The model under review builds one solid part; all positions refer to its coordinate system, in mm. A direction names the side the tool comes from. Coordinates: 2 decimals unless noted, no trailing zeros. Order: outer loops, then holes, each group sorted by start corner. A loop starts at its lowest first (then second) coordinate and runs counter-clockwise, first axis right, second up. Notation, with made-up numbers: M -30.5,70.25 L 28.5,70.25 A23 cw 28.5,98.25 Z; hole C 61,24.25 d4. An arc over 180 degrees is marked long. One line per item, written item: value.
Autodesk Inventor part; units mm, degrees
ref_plane "YZ Plane" through (0, 0, 0) normal (1, 0, 0) x (0, 1, 0)
ref_plane "XZ Plane" through (0, 0, 0) normal (0, 1, 0) x (-1, 0, 0)
ref_plane "XY Plane" through (0, 0, 0) normal (0, 0, 1) x (1, 0, 0)
sketch "Sketch1" plane through (0, 0, 0) normal (0, 1, 0) x (-1, 0, 0)
  line L0 (76.2, -76.2) -> (-76.2, -76.2)
  line L1 (-76.2, -76.2) -> (-76.2, 76.2)
  line L2 (76.2, 76.2) -> (76.2, -76.2)
  line L3 (-22.225, -25.4) -> (22.225, -25.4)
  line L4 (22.225, -25.4) -> (22.225, -69.85)
  line L5 (22.225, -69.85) -> (-22.225, -69.85)
  line L6 (-22.225, -69.85) -> (-22.225, -25.4)
  line L7 (-19.05, 56.2) -> (19.05, 56.2)
  line L8 (-76.2, 76.2) -> (-39.05, 76.2)
  line L9 (39.05, 76.2) -> (76.2, 76.2)
  line L10 (19.05, 56.2) -> (39.05, 76.2)
  line L11 (-19.05, 56.2) -> (-39.05, 76.2)
  point P0 (0, 0)
  dimension "d0" = 152.4
  dimension "d2" = 152.4
  dimension "d3" = 76.2
  dimension "d4" = 76.2
  dimension "d5" = 44.45
  dimension "d6" = 44.45
  dimension "d7" = 22.225
  dimension "d26" = 56.2
  dimension "d31" = 45
  dimension "d32" = 45
  dimension "d33" = 38.1
  dimension "d34" = 57.15
  dimension "d56" = 6.35
extrude "Extrusion1" add sketch "Sketch1" along normal blind 6.35
chamfer "Chamfer2" distance 3.175 angle 45 1 edges at (76.2, 3.175, 76.2)
chamfer "Chamfer3" distance 3.175 angle 45 3 edges at (76.2, 3.175, -76.2) (-76.2, 3.175, -76.2) (-76.2, 3.175, 76.2)
sketch "Sketch3" plane through (0, 6.35, 0) normal (0, 1, 0) x (1, 0, 0)
  line L0 (-18.415, 21.59) -> (18.415, 21.59)
  line L1 (21.59, 18.415) -> (21.59, -18.415)
  line L2 (18.415, -21.59) -> (-18.415, -21.59)
  line L3 (-21.59, -18.415) -> (-21.59, 18.415)
  line L4 (-21.59, 18.415) -> (-18.415, 21.59)
  line L5 (18.415, 21.59) -> (21.59, 18.415)
  line L6 (21.59, -18.415) -> (18.415, -21.59)
  line L7 (-18.415, -21.59) -> (-21.59, -18.415)
  point P0 (0, 0)
  point P1 (-21.59, 21.59)
  point P2 (21.59, -21.59)
  point P3 (21.59, 21.59)
  point P4 (-21.59, -21.59)
  dimension "d41" = 43.18
  dimension "d43" = 43.18
  dimension "d44" = 21.59
  dimension "d45" = 21.59
  dimension "d46" = 3.175
  dimension "d47" = 3.175
  dimension "d48" = 3.175
  dimension "d49" = 3.175
  dimension "d50" = 3.175
  dimension "d51" = 3.175
  dimension "d52" = 3.175
  dimension "d53" = 3.175
extrude "Extrusion2" cut sketch "Sketch3" against normal through all
chamfer "Chamfer4" distance 3.175 angle 45 4 edges at (-22.225, 3.175, -69.85) (-22.225, 3.175, -25.4) (22.225, 3.175, -69.85) (22.225, 3.175, -25.4)
sketch "Sketch4" plane through (0, 6.35, 0) normal (0, 1, 0) x (1, 0, 0)
  line L0 (73.025, 76.2) -> (-73.025, 76.2)
  line L1 (-76.2, 73.025) -> (-76.2, -73.025)
  line L2 (-66.675, 69.85) -> (-43.815, 69.85)
  line L3 (-43.815, 69.85) -> (-43.815, 57.785)
  line L4 (-43.815, 57.785) -> (-66.675, 57.785)
  line L5 (-66.675, 57.785) -> (-66.675, 69.85)
  point P0 (0, 0)
  dimension "d60" = 12.065
  dimension "d62" = 22.86
  dimension "d65" = 9.525
  dimension "d66" = 6.35
extrude "Extrusion3" cut sketch "Sketch4" against normal through all
equation "\"d34\" = -0.5 * d33 + 0.5 * d0"
properties part number "carousel_base"
(1) We need section B-B, the plane y = 3.5. Count the separate pieces of the cut face and the enclosed holes in it, plus the area to 3 significant figures.
Geometry results:
separate pieces: 1
enclosed holes: 3
area: 18,000 mm2
(2) For L1, parallel to X at y = 0.5, z = -63.5 (3 decimals); L2, parallel to Z at x = 10, y = 1.25; L3, parallel to Z at x = -55.5, y = 1.75 (3 decimals), list the stretches that pass through material, from the lowest coordinate up.
Geometry results:
L1: x = -76.2 to -66.675, -43.815 to -22.225, 22.225 to 76.2
L2: z = -76.2 to -69.85, -25.4 to -21.59, 21.59 to 56.2
L3: z = -76.2 to -69.85, -57.785 to 76.2
(3) Mouldability with a two-part tool opening along Z and no side actions: class faces 1 (the flat face through (-1, 3, -76.2)), 2 (the flat face through (0, 3, -69.85)), 3 (the flat face through (56, 3, 76.2)) as +Z half, -Z half, draft (parallel to the pull), parting line (faces both ways), or undercut.
Geometry results:
face 1: -Z half
face 2: undercut
face 3: +Z half
(4) We need section D-D, the plane z = 5. State the section outline as (x, y) points.
Geometry results:
outline: M -76.2,0 L -21.59,0 L -21.59,6.35 L -76.2,6.35 Z; M 21.59,0 L 76.2,0 L 76.2,6.35 L 21.59,6.35 Z
(5) Insertion check: pin 1 Ø1.9 at (x, y) = (8.5, 2) entering from +Z. The pin has a flat end and moves straight along its axis. Give the tip position at first contact, or say it passes through.
Geometry results:
pin 1: stops at z = 56.2
(6) We need section C-C, the plane x = 30.5. State the section outline as (y, z) points, plus the area to 3 significant figures.
Geometry results:
outline: M 0,-76.2 L 6.35,-76.2 L 6.35,67.65 L 0,67.65 Z
area: 913 mm2
(7) We need section A-A, the plane z = 63.5. State the section outline as (x, y) points, plus the area to 3 significant figures.
Geometry results:
outline: M -76.2,0 L -26.35,0 L -26.35,6.35 L -76.2,6.35 Z; M 26.35,0 L 76.2,0 L 76.2,6.35 L 26.35,6.35 Z
area: 633 mm2
(8) Tool access review of faces 4 (the flat face through (-66.675, 3, -64)), 5 (the flat face through (-56, 3, 76.2)), 6 (the flat face through (0, 3, 56.2)): name each direction out of +Z, -Z, +X, -X, +Y, -Y from which nothing blocks a thin tool from reaching the whole face with its end or side.
Geometry results:
face 4: +Y, -Y
face 5: +Z, +X, -X, +Y, -Y
face 6: +Z, +Y, -Y
